Could you check a few things on this model? Use its own coordinates, in mm. Round coordinates to 2 decimals unless told otherwise and drop trailing zeros. Order: outer loops, then holes, each group sorted by start corner. A loop starts at its lowest first (then second) coordinate and runs counter-clockwise, first axis right, second up. Notation, with made-up numbers: M 2,50.5 L 26,50.5 A20 cw 26,73.5 Z; hole C 75,32.25 d4. An arc over 180 degrees is marked long. Write each question's results on one line, items separated by ' | '. Start each with the question number.
1. Please list where these lines run through material, in increasing order: L1, parallel to X at y = 0.8, z = -63; L2, parallel to X at y = 2.3, z = 92; L3, parallel to Z at x = 50, y = 2.45.
2. Suppose I cut it at A-A on x = 67.5. Write out the boundary of the cut face in (y, z).
3. Suppose I cut it at B-B on y = 1.75. Give the number of separate pieces and of enclosed holes in the cut face, and give its area (3 significant figures).
4. Suppose I cut it at D-D on x = 113.5. Write out the boundary of the cut face in (y, z).
5. I'm going to push flat-ended pins straight in: pin 1 (1.5 mm diameter, centred on y = 1, z = 3, fed in from -X); pin 2 (4 mm diameter, centred on x = 117, z = -72.29, fed in from +Y); pin 3 (0.9 mm diameter, centred on x = 118.5, y = 1.5, fed in from +Z); pin 4 (1.5 mm diameter, centred on y = 1.5, z = -22.5, fed in from -X). Where does each tip first touch, or does it pass through?
6. Suppose I cut it at C-C on z = 87. Write out the boundary of the cut face in (x, y).
from build123d import *

# Parameters (mm, degrees)
BOSS_EXTRUDE1_DEPTH = 3
CUT_EXTRUDE1_REACH  = 162.106
SKETCH2_W           = 45
SKETCH2_H           = 74
FILLET2_R           = 3
SKETCH3_W           = 3.1
SKETCH3_H           = 10.1
CUT_EXTRUDE2_DEPTH  = 161.106214745
CUT_EXTRUDE3_REACH  = 162.106
SKETCH4_R           = 1.6
SKETCH5_R           = 3.5
CUT_EXTRUDE4_DEPTH  = 161.106214745


with BuildPart() as part:
    # Sketch1 → Boss-Extrude1 (new body)
    with BuildSketch(Plane(origin=(0, 0, 0), x_dir=(1, 0, 0), z_dir=(0, 1, 0))):
        Polygon((42.5, 100), (85, 100), (125, 76.905989232), (125, -76.905989232), (85, -100), (42.5, -100), align=None)
        with BuildLine():
            Line((99.3, 23), (67.3, 23))
            ThreePointArc((67.3, 23), (63.764466094, 21.535533906), (62.3, 18))
            Line((62.3, 18), (62.3, -14))
            ThreePointArc((62.3, -14), (63.764466094, -17.535533906), (67.3, -19))
            Line((67.3, -19), (99.3, -19))
            ThreePointArc((99.3, -19), (102.835533906, -17.535533906), (104.3, -14))
            Line((104.3, -14), (104.3, 18))
            ThreePointArc((104.3, 18), (102.835533906, 21.535533906), (99.3, 23))
        make_face(mode=Mode.SUBTRACT)
    extrude(amount=BOSS_EXTRUDE1_DEPTH)

    # Sketch2 → Cut-Extrude1 (cut, up to next)
    with BuildSketch(Plane(origin=(0, 3, 0), x_dir=(1, 0, 0), z_dir=(0, 1, 0)), mode=Mode.PRIVATE) as cut_extrude1_sk1:
        with Locations((65, 18)):
            Rectangle(SKETCH2_W, SKETCH2_H)
    cut_extrude1_tool1 = extrude(cut_extrude1_sk1.sketch, amount=-CUT_EXTRUDE1_REACH, mode=Mode.PRIVATE) & part.part
    add(cut_extrude1_tool1.solids().sort_by_distance((65, 3, -18))[0], mode=Mode.SUBTRACT)

    # Fillet2
    fillet2_edges = [part.edges().sort_by_distance(p)[0] for p in [
        (125, 1.5, -76.905989232),
        (125, 1.5, 76.905989232),
        (85, 1.5, 100),
        (42.5, 1.5, 100),
        (42.5, 1.5, -100),
        (85, 1.5, -100),
        (42.5, 1.5, 19),
        (42.5, 1.5, -55),
        (87.5, 1.5, -23),
        (87.5, 1.5, -55),
    ]]
    fillet(fillet2_edges, radius=FILLET2_R)

    # Sketch3 → Cut-Extrude2 (cut, through all)
    with BuildSketch(Plane(origin=(0, 3, 0), x_dir=(1, 0, 0), z_dir=(0, 1, 0))):
        with Locations((118.45, 20)):
            Rectangle(SKETCH3_W, SKETCH3_H)
        with Locations((118.45, -20)):
            Rectangle(SKETCH3_W, SKETCH3_H)
        with Locations((118.45, 60)):
            Rectangle(SKETCH3_W, SKETCH3_H)
        with Locations((118.45, -60)):
            Rectangle(SKETCH3_W, SKETCH3_H)
    extrude(amount=-CUT_EXTRUDE2_DEPTH, mode=Mode.SUBTRACT)

    # Sketch4 → Cut-Extrude3 (cut, up to next)
    with BuildSketch(Plane(origin=(0, 3, 0), x_dir=(1, 0, 0), z_dir=(0, 1, 0)), mode=Mode.PRIVATE) as cut_extrude3_sk1:
        with Locations(Location((50.5, 92, 0), (0, 0, 270))):
            Circle(SKETCH4_R)
    cut_extrude3_tool1 = extrude(cut_extrude3_sk1.sketch, amount=-CUT_EXTRUDE3_REACH, mode=Mode.PRIVATE) & part.part
    # Sketch4 → Cut-Extrude3 (cut, up to next)
    with BuildSketch(Plane(origin=(0, 3, 0), x_dir=(1, 0, 0), z_dir=(0, 1, 0)), mode=Mode.PRIVATE) as cut_extrude3_sk2:
        with Locations(Location((50.5, 63, 0), (0, 0, 270))):
            Circle(SKETCH4_R)
    cut_extrude3_tool2 = extrude(cut_extrude3_sk2.sketch, amount=-CUT_EXTRUDE3_REACH, mode=Mode.PRIVATE) & part.part
    # Sketch4 → Cut-Extrude3 (cut, up to next)
    with BuildSketch(Plane(origin=(0, 3, 0), x_dir=(1, 0, 0), z_dir=(0, 1, 0)), mode=Mode.PRIVATE) as cut_extrude3_sk3:
        with Locations(Location((50.5, -60, 0), (0, 0, 270))):
            Circle(SKETCH4_R)
    cut_extrude3_tool3 = extrude(cut_extrude3_sk3.sketch, amount=-CUT_EXTRUDE3_REACH, mode=Mode.PRIVATE) & part.part
    # Sketch4 → Cut-Extrude3 (cut, up to next)
    with BuildSketch(Plane(origin=(0, 3, 0), x_dir=(1, 0, 0), z_dir=(0, 1, 0)), mode=Mode.PRIVATE) as cut_extrude3_sk4:
        with Locations(Location((50.5, -92, 0), (0, 0, 270))):
            Circle(SKETCH4_R)
    cut_extrude3_tool4 = extrude(cut_extrude3_sk4.sketch, amount=-CUT_EXTRUDE3_REACH, mode=Mode.PRIVATE) & part.part
    # Sketch4 → Cut-Extrude3 (cut, up to next)
    with BuildSketch(Plane(origin=(0, 3, 0), x_dir=(1, 0, 0), z_dir=(0, 1, 0)), mode=Mode.PRIVATE) as cut_extrude3_sk5:
        with Locations(Location((117, 72.287187079, 0), (0, 0, 270))):
            Circle(SKETCH4_R)
    cut_extrude3_tool5 = extrude(cut_extrude3_sk5.sketch, amount=-CUT_EXTRUDE3_REACH, mode=Mode.PRIVATE) & part.part
    # Sketch4 → Cut-Extrude3 (cut, up to next)
    with BuildSketch(Plane(origin=(0, 3, 0), x_dir=(1, 0, 0), z_dir=(0, 1, 0)), mode=Mode.PRIVATE) as cut_extrude3_sk6:
        with Locations(Location((117, -72.287187079, 0), (0, 0, 270))):
            Circle(SKETCH4_R)
    cut_extrude3_tool6 = extrude(cut_extrude3_sk6.sketch, amount=-CUT_EXTRUDE3_REACH, mode=Mode.PRIVATE) & part.part
    # Sketch4 → Cut-Extrude3 (cut, up to next)
    with BuildSketch(Plane(origin=(0, 3, 0), x_dir=(1, 0, 0), z_dir=(0, 1, 0)), mode=Mode.PRIVATE) as cut_extrude3_sk7:
        with Locations(Location((82.856406461, 92, 0), (0, 0, 270))):
            Circle(SKETCH4_R)
    cut_extrude3_tool7 = extrude(cut_extrude3_sk7.sketch, amount=-CUT_EXTRUDE3_REACH, mode=Mode.PRIVATE) & part.part
    # Sketch4 → Cut-Extrude3 (cut, up to next)
    with BuildSketch(Plane(origin=(0, 3, 0), x_dir=(1, 0, 0), z_dir=(0, 1, 0)), mode=Mode.PRIVATE) as cut_extrude3_sk8:
        with Locations(Location((82.856406461, -92, 0), (0, 0, 270))):
            Circle(SKETCH4_R)
    cut_extrude3_tool8 = extrude(cut_extrude3_sk8.sketch, amount=-CUT_EXTRUDE3_REACH, mode=Mode.PRIVATE) & part.part
    add(cut_extrude3_tool1.solids().sort_by_distance((50.5, 3, -92))[0], mode=Mode.SUBTRACT)
    add(cut_extrude3_tool2.solids().sort_by_distance((50.5, 3, -63))[0], mode=Mode.SUBTRACT)
    add(cut_extrude3_tool3.solids().sort_by_distance((50.5, 3, 60))[0], mode=Mode.SUBTRACT)
    add(cut_extrude3_tool4.solids().sort_by_distance((50.5, 3, 92))[0], mode=Mode.SUBTRACT)
    add(cut_extrude3_tool5.solids().sort_by_distance((117, 3, -72.287187))[0], mode=Mode.SUBTRACT)
    add(cut_extrude3_tool6.solids().sort_by_distance((117, 3, 72.287187))[0], mode=Mode.SUBTRACT)
    add(cut_extrude3_tool7.solids().sort_by_distance((82.856406, 3, -92))[0], mode=Mode.SUBTRACT)
    add(cut_extrude3_tool8.solids().sort_by_distance((82.856406, 3, 92))[0], mode=Mode.SUBTRACT)

    # Sketch5 → Cut-Extrude4 (cut, through all)
    with BuildSketch(Plane(origin=(0, 3, 0), x_dir=(1, 0, 0), z_dir=(0, 1, 0))):
        with Locations(Location((67.5, 75, 0), (0, 0, 270))):
            Circle(SKETCH5_R)
        with Locations(Location((67.5, -75, 0), (0, 0, 90))):
            Circle(SKETCH5_R)
    extrude(amount=-CUT_EXTRUDE4_DEPTH, mode=Mode.SUBTRACT)


solid = part.part
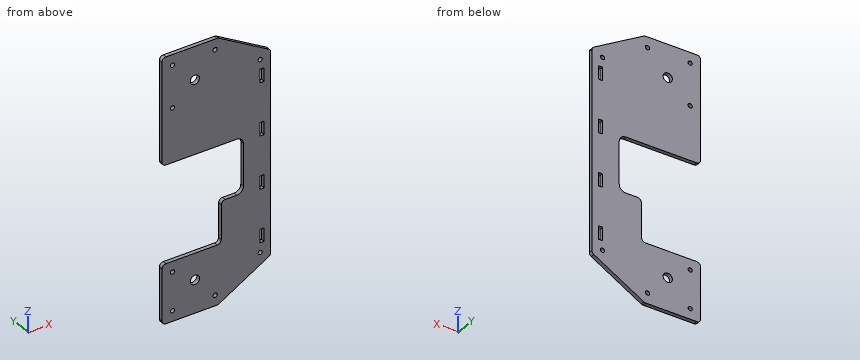
Filled sheet:
1) L1: x = 42.5 to 48.9, 52.1 to 116.9, 120 to 125 | L2: x = 42.5 to 48.9, 52.1 to 81.26, 84.46 to 98.86 | L3: z = -100 to -93.52, -90.48 to -64.52, -61.48 to -55, 19 to 58.48, 61.52 to 90.48, 93.52 to 100
2) outline: M 0,-100 L 3,-100 L 3,-78.5 L 0,-78.5 Z; M 0,-71.5 L 3,-71.5 L 3,-55 L 0,-55 Z; M 0,19 L 3,19 L 3,71.5 L 0,71.5 Z; M 0,78.5 L 3,78.5 L 3,100 L 0,100 Z
3) separate pieces: 1 | enclosed holes: 14 | area: 11,300 mm^2
4) outline: M 0,-83.55 L 3,-83.55 L 3,83.55 L 0,83.55 Z
5) pin 1: stops at x = 104.3 | pin 2: stops at y = 3 | pin 3: stops at z = 80.92 | pin 4: stops at x = 89.3
6) outline: M 42.5,0 L 107.52,0 L 107.52,3 L 42.5,3 Z
